Autodesk Inventor part; units mm, degrees
ref_plane "YZ Plane" through (0, 0, 0) normal (1, 0, 0) x (0, 1, 0)
ref_plane "XZ Plane" through (0, 0, 0) normal (0, 1, 0) x (-1, 0, 0)
ref_plane "XY Plane" through (0, 0, 0) normal (0, 0, 1) x (1, 0, 0)
sketch "Sketch1" plane through (0, 0, 0) normal (0, 0, 1) x (1, 0, 0)
  line L0 (-10, 10) -> (10, 10) construction
  line L1 (10, 10) -> (10, -10) construction
  line L2 (10, -10) -> (-10, -10) construction
  line L3 (-10, -10) -> (-10, 10) construction
  line L4 (-10, 10) -> (10, -10) construction
  line L5 (10, 10) -> (-10, -10) construction
  circle A0 centre (0, 0) radius 2
  line L6 (-4, -4) -> (4, -4) construction
  line L7 (4, -4) -> (4, 4) construction
  line L8 (4, 4) -> (-4, 4) construction
  line L9 (-4, 4) -> (-4, -4) construction
  line L10 (-4, -4) -> (4, 4) construction
  line L11 (4, -4) -> (-4, 4) construction
  line L12 (2.6444, 4.0586) -> (6.2444, 7.6586)
  line L13 (6.1029, 8) -> (3.3, 8)
  line L14 (3.1, 8.2) -> (3.1, 9.8)
  line L15 (3.3, 10) -> (8.5, 10)
  line L16 (4.0586, 2.6444) -> (7.6586, 6.2444)
  line L17 (8, 6.1029) -> (8, 3.3)
  line L18 (8.2, 3.1) -> (9.8, 3.1)
  line L19 (10, 8.5) -> (10, 3.3)
  line L20 (0, 4) -> (2.5029, 4)
  line L21 (4, 0) -> (4, 2.5029)
  line L22 (0, 10) -> (0, -10) construction
  line L23 (-10, 0) -> (10, 0) construction
  line L24 (-2.6444, 4.0586) -> (-6.2444, 7.6586)
  line L25 (-6.1029, 8) -> (-3.3, 8)
  line L26 (-3.1, 8.2) -> (-3.1, 9.8)
  line L27 (-3.3, 10) -> (-8.5, 10)
  line L28 (-4.0586, 2.6444) -> (-7.6586, 6.2444)
  line L29 (-8, 6.1029) -> (-8, 3.3)
  line L30 (-8.2, 3.1) -> (-9.8, 3.1)
  line L31 (-10, 8.5) -> (-10, 3.3)
  line L32 (0, 4) -> (-2.5029, 4)
  line L33 (-4, 0) -> (-4, 2.5029)
  line L34 (2.6444, -4.0586) -> (6.2444, -7.6586)
  line L35 (6.1029, -8) -> (3.3, -8)
  line L36 (3.1, -8.2) -> (3.1, -9.8)
  line L37 (3.3, -10) -> (8.5, -10)
  line L38 (4.0586, -2.6444) -> (7.6586, -6.2444)
  line L39 (8, -6.1029) -> (8, -3.3)
  line L40 (8.2, -3.1) -> (9.8, -3.1)
  line L41 (10, -8.5) -> (10, -3.3)
  line L42 (0, -4) -> (2.5029, -4)
  line L43 (4, 0) -> (4, -2.5029)
  line L44 (0, -4) -> (-2.5029, -4)
  line L45 (-2.6444, -4.0586) -> (-6.2444, -7.6586)
  line L46 (-6.1029, -8) -> (-3.3, -8)
  line L47 (-3.1, -8.2) -> (-3.1, -9.8)
  line L48 (-3.3, -10) -> (-8.5, -10)
  line L49 (-4.0586, -2.6444) -> (-7.6586, -6.2444)
  line L50 (-4, 0) -> (-4, -2.5029)
  line L51 (-8, -6.1029) -> (-8, -3.3)
  line L52 (-8.2, -3.1) -> (-9.8, -3.1)
  line L53 (-10, -8.5) -> (-10, -3.3)
  arc A1 (10, 8.5) -> (8.5, 10) centre (8.5, 8.5) ccw
  arc A2 (-8.5, 10) -> (-10, 8.5) centre (-8.5, 8.5) ccw
  arc A3 (-10, -8.5) -> (-8.5, -10) centre (-8.5, -8.5) ccw
  arc A4 (8.5, -10) -> (10, -8.5) centre (8.5, -8.5) ccw
  arc A5 (-3.1, 9.8) -> (-3.3, 10) centre (-3.3, 9.8) ccw
  arc A6 (-3.3, 8) -> (-3.1, 8.2) centre (-3.3, 8.2) ccw
  arc A7 (-6.1029, 8) -> (-6.2444, 7.6586) centre (-6.1029, 7.8) ccw
  arc A8 (6.2444, 7.6586) -> (6.1029, 8) centre (6.1029, 7.8) ccw
  arc A9 (-8, -6.1029) -> (-7.6586, -6.2444) centre (-7.8, -6.1029) ccw
  arc A10 (-3.1, -8.2) -> (-3.3, -8) centre (-3.3, -8.2) ccw
  arc A11 (6.1029, -8) -> (6.2444, -7.6586) centre (6.1029, -7.8) ccw
  arc A12 (3.3, -8) -> (3.1, -8.2) centre (3.3, -8.2) ccw
  arc A13 (-6.2444, -7.6586) -> (-6.1029, -8) centre (-6.1029, -7.8) ccw
  arc A14 (7.6586, -6.2444) -> (8, -6.1029) centre (7.8, -6.1029) ccw
  arc A15 (8.2, -3.1) -> (8, -3.3) centre (8.2, -3.3) ccw
  arc A16 (8, 6.1029) -> (7.6586, 6.2444) centre (7.8, 6.1029) ccw
  arc A17 (8, 3.3) -> (8.2, 3.1) centre (8.2, 3.3) ccw
  arc A18 (3.3, 10) -> (3.1, 9.8) centre (3.3, 9.8) ccw
  arc A19 (-2.6444, 4.0586) -> (-2.5029, 4) centre (-2.5029, 4.2) ccw
  arc A20 (2.5029, 4) -> (2.6444, 4.0586) centre (2.5029, 4.2) ccw
  arc A21 (4.0586, 2.6444) -> (4, 2.5029) centre (4.2, 2.5029) ccw
  arc A22 (4, -2.5029) -> (4.0586, -2.6444) centre (4.2, -2.5029) ccw
  arc A23 (2.6444, -4.0586) -> (2.5029, -4) centre (2.5029, -4.2) ccw
  arc A24 (-2.5029, -4) -> (-2.6444, -4.0586) centre (-2.5029, -4.2) ccw
  arc A25 (-4.0586, -2.6444) -> (-4, -2.5029) centre (-4.2, -2.5029) ccw
  arc A26 (-4, 2.5029) -> (-4.0586, 2.6444) centre (-4.2, 2.5029) ccw
  arc A27 (-7.6586, 6.2444) -> (-8, 6.1029) centre (-7.8, 6.1029) ccw
  arc A28 (-8.2, 3.1) -> (-8, 3.3) centre (-8.2, 3.3) ccw
  arc A29 (-10, 3.3) -> (-9.8, 3.1) centre (-9.8, 3.3) ccw
  arc A30 (-8, -3.3) -> (-8.2, -3.1) centre (-8.2, -3.3) ccw
  arc A31 (-9.8, -3.1) -> (-10, -3.3) centre (-9.8, -3.3) ccw
  arc A32 (-3.3, -10) -> (-3.1, -9.8) centre (-3.3, -9.8) ccw
  arc A33 (3.1, -9.8) -> (3.3, -10) centre (3.3, -9.8) ccw
  arc A34 (10, -3.3) -> (9.8, -3.1) centre (9.8, -3.3) ccw
  arc A35 (9.8, 3.1) -> (10, 3.3) centre (9.8, 3.3) ccw
  arc A36 (3.1, 8.2) -> (3.3, 8) centre (3.3, 8.2) ccw
  point P0 (2.5858, 4)
  point P1 (6.5858, 8)
  point P2 (3.1, 8)
  point P3 (3.1, 10)
  point P4 (4, 2.5858)
  point P5 (8, 6.5858)
  point P6 (8, 3.1)
  point P7 (10, 3.1)
  point P8 (-2.5858, 4)
  point P9 (-6.5858, 8)
  point P10 (-3.1, 8)
  point P11 (-3.1, 10)
  point P12 (-4, 2.5858)
  point P13 (-8, 6.5858)
  point P14 (-8, 3.1)
  point P15 (-10, 3.1)
  point P16 (2.5858, -4)
  point P17 (6.5858, -8)
  point P18 (3.1, -8)
  point P19 (3.1, -10)
  point P20 (4, -2.5858)
  point P21 (8, -6.5858)
  point P22 (8, -3.1)
  point P23 (10, -3.1)
  point P24 (-2.5858, -4)
  point P25 (-6.5858, -8)
  point P26 (-3.1, -8)
  point P27 (-3.1, -10)
  point P28 (-4, -2.5858)
  point P29 (-8, -6.5858)
  point P30 (-8, -3.1)
  point P31 (-10, -3.1)
  dimension "d0" = 20
  dimension "d1" = 20
  dimension "d2" = 4
  dimension "d5" = 6
  dimension "t" = 2
  dimension "d7" = 1
  dimension "d8" = 2
  dimension "d9" = 2
  dimension "d10" = 3.1
  dimension "d11" = 3.1
  dimension "d15" = 1.5
  dimension "d16" = 1.5
  dimension "d17" = 1.5
  dimension "d18" = 1.5
  dimension "d19" = 0.2
  dimension "d20" = 0.2
  dimension "d21" = 0.2
  dimension "d22" = 0.2
  dimension "d23" = 0.2
  dimension "d24" = 0.2
  dimension "d25" = 0.2
  dimension "d26" = 0.2
  dimension "d27" = 0.2
  dimension "d28" = 0.2
  dimension "d29" = 0.2
  dimension "d30" = 0.2
  dimension "d31" = 0.2
  dimension "d32" = 0.2
  dimension "d33" = 0.2
  dimension "d34" = 0.2
  dimension "d35" = 0.2
  dimension "d36" = 0.2
  dimension "d37" = 0.2
  dimension "d38" = 0.2
  dimension "d39" = 0.2
  dimension "d40" = 0.2
  dimension "d41" = 0.2
extrude "2020 Al T-S (1000mm)" add sketch "Sketch1" along normal blind 152.4
equation "\"d1\" = d0"
equation "\"d7\" = 0.5 * t"
equation "\"d8\" = t"
equation "\"d9\" = t"
equation "\"d11\" = d10"
properties part number "2020 Aluminium Extrusion T-Slot" material "Aluminum 6061"
The listing builds one solid part. Answer for the finished solid, in the listing's coordinates (mm). A direction names the side the tool comes from. Give positions to 0.01 mm unless a question says otherwise; leave off trailing zeros. Write each loop counter-clockwise with the first axis right and the second up, starting at its lowest first coordinate (ties: lowest second). Pieces come first, ordered by that corner, then holes. Notation, with made-up numbers: (-6, -18.75) - (2, -18.75) arc R18 cw to (2, 16.25) - close; hole circle Ø5 at (-16, 32.25). An arc over 180 degrees is marked (long way). Use one line per item in the form item = value. Start each with the question number.
1) Find section A-A on x = 0. Determine the outline of the cut face in (y, z), plus the area to 3 significant figures.
2) Consider line 1 along X through (y, z) = (6, 18.5); line 2 along Y through (x, z) = (0, 52.5); line 3 along X through (y, z) = (-7.75, 18). Determine where each line is inside the solid, lowest interval first. Write a range as from..to.
3) Flat-ended cylindrical pins translate along their axes: pin 1 Ø1.5 at (x, z) = (1, 97.5) entering from -Y; pin 2 Ø4 at (y, z) = (-0.5, 109.5) entering from -X; pin 3 Ø0.5 at (y, z) = (-9, 39) entering from -X. Find the tip coordinate at first contact, or state that the pin passes through.
4) The mould has two halves that part along X. Classify faces 5 (the face through (8, -5, 75)), 6 (the face through (-10, 6, 75)), 7 (the face through (4, 0, 75)): pulls with the +X half, pulls with the -X half, needs draft (parallel to the pull), parting line crosses it, or undercut.
5) A tool of negligible diameter and unlimited length cuts with its end or side. For faces 1 (the face through (0, -4, 75)), 2 (the face through (-10, -6, 75)), 3 (the face through (0, 4, 75)), 4 (the face through (5.833, 4.419, 75.133)), from which of +Z, -Z, +X, -X, +Y, -Y can it reach the whole face along a straight path? Write none if from no direction.
Geometry results:
q1.outline = (-4, 0) - (-2, 0) - (-2, 152.4) - (-4, 152.4) - close; (2, 0) - (4, 0) - (4, 152.4) - (2, 152.4) - close
q1.area = 610 mm2
q2.line_1 = -10..-8, -7.41..-4.59, 4.59..7.41, 8..10
q2.line_2 = -4..-2, 2..4
q2.line_3 = -10..-6.3, 6.3..10
q3.pin_1 = -4
q3.pin_2 = -4
q3.pin_3 = -9.98
q4.face_5 = undercut
q4.face_6 = pulls with the -X half
q4.face_7 = pulls with the +X half
q5.face_1 = +Z, -Z, -Y
q5.face_2 = +Z, -Z, -X, +Y, -Y
q5.face_3 = +Z, -Z, +Y
q5.face_4 = +Z, -Z
